Here's how the part is built. I have some questions about the finished solid (model axes, mm). Round coordinates to 2 decimals unless told otherwise and drop trailing zeros. Write each loop counter-clockwise with the first axis right and the second up, starting at its lowest first coordinate (ties: lowest second). Pieces come first, ordered by that corner, then holes. Notation, with made-up numbers: M -16,20.25 L 10,20.25 A8 cw 10,28.25 Z; hole C -18,49.25 d9. An arc over 180 degrees is marked long. Use one line per item in the form item = value. Start each with the question number.
Q1. I need wall thicknesses on line 1 along X through (y, z) = (0.25, 5); line 2 along X through (y, z) = (0.4, 16); line 3 along Z through (x, y) = (1.5, 0.2). Which ranges of each line are inside material? Lowest first, please. Write a range as from..to.
Q2. I want a section at A-A on y = 0.65. List the corners of the cut face in (x, z) for me.
Q3. We'd pull the mould along Z, two halves only. Please class faces 1 (the face through (14.4, 0.5, 20)), 2 (the face through (14.4, 0.5, 0)), 3 (the face through (26.272, 0.507, 16.364)), 4 (the face through (31.338, 0.5, 10.1)): +Z half, -Z half, draft (parallel to the pull), parting line (faces both ways), or undercut.
Q4. I'm going to push a flat-ended pin straight in: pin 1 Ø2.5 at (x, z) = (26.58, 5) entering from +Y. Where does the tip first touch, or does it pass through?
Q5. I want a section at B-B on z = 15. List the corners of the cut face in (x, y) for me, and give its area (3 significant figures).
```python
from build123d import *

# Parameters (mm, degrees)
BOSS_EXTRUDE1_DEPTH = 20
SKETCH6_R           = 1.397
CUT_EXTRUDE1_DEPTH  = 1
SKETCH7_W           = 2.16646989
SKETCH7_H           = 20
BOSS_EXTRUDE2_DEPTH = 1


with BuildPart() as part:
    # Sketch1 → Boss-Extrude1 (new body)
    with BuildSketch(Plane.XY):
        Polygon((0, 0), (2.596030114, 0), (29.171217845, 0), (29.171217845, 1), (26.575187731, 1), (0, 1), align=None)
    extrude(amount=BOSS_EXTRUDE1_DEPTH)

    # Sketch6 → Cut-Extrude1 (cut)
    with BuildSketch(Plane(origin=(0, 1, 0), x_dir=(1, 0, 0), z_dir=(0, 1, 0))):
        with Locations((26.575187731, -15.000000033)):
            Circle(SKETCH6_R)
        with Locations((2.596030114, -15.000000033)):
            Circle(SKETCH6_R)
        with Locations((2.596030114, -4.999999967)):
            Circle(SKETCH6_R)
        with Locations((26.575187731, -4.999999967)):
            Circle(SKETCH6_R)
    extrude(amount=-CUT_EXTRUDE1_DEPTH, mode=Mode.SUBTRACT)

    # Sketch7 → Boss-Extrude2 (add)
    with BuildSketch(Plane(origin=(0, 1, 0), x_dir=(1, 0, 0), z_dir=(0, 1, 0))):
        with Locations((30.25445279, -10)):
            Rectangle(SKETCH7_W, SKETCH7_H)
        with Locations((-1.083234945, -10)):
            Rectangle(SKETCH7_W, SKETCH7_H)
    extrude(amount=-BOSS_EXTRUDE2_DEPTH)


solid = part.part
```
Reported:
q1.line_1 = -2.17..1.2, 3.99..25.18, 27.97..31.34
q1.line_2 = -2.17..1.62, 3.57..25.6, 27.55..31.34
q1.line_3 = 0..4.13, 5.87..14.13, 15.87..20
q2.outline = M -2.17,0 L 31.34,0 L 31.34,20 L -2.17,20 Z; hole C 2.6,5 d2.79; hole C 2.6,15 d2.79; hole C 26.58,5 d2.79; hole C 26.58,15 d2.79
q3.face_1 = +Z half
q3.face_2 = -Z half
q3.face_3 = undercut
q3.face_4 = draft
q4.pin_1 = through
q5.outline = M -2.17,0 L 1.2,0 L 1.2,1 L -2.17,1 Z; M 3.99,0 L 25.18,0 L 25.18,1 L 3.99,1 Z; M 27.97,0 L 31.34,0 L 31.34,1 L 27.97,1 Z
q5.area = 27.9 mm^2
